Autodesk Inventor part; units mm, degrees
ref_plane "XZ Plane" through (0, 0, 0) normal (0, 1, 0) x (-1, 0, 0)
ref_plane "XY Plane" through (0, 0, 0) normal (0, 0, 1) x (1, 0, 0)
sketch "Sketch1" plane through (0, 0, 0) normal (0, 1, 0) x (-1, 0, 0)
  line L0 (0, 0) -> (60, 0)
  line L1 (60, 0) -> (60, -120)
  line L2 (60, -120) -> (0, -120)
  line L3 (0, -120) -> (0, 0)
  line L4 (60, 0) -> (0, -120) construction
  line L5 (60, -120) -> (0, 0) construction
  circle A0 centre (30, -60) radius 67.082
  line L6 (30, -120) -> (30, 7.082) construction
  line L7 (60, -60) -> (0, -60)
  line L8 (30, -60) -> (81.3878, -103.1195) construction
  line L9 (41.76, -45.985) -> (17.4815, -74.919) construction
  line L10 (-33, -36.9566) -> (-33, -83.0434)
  line L11 (93, -36.9566) -> (93, -83.0434)
  circle A1 centre (60, -110) radius 1.5
  circle A2 centre (70, -60) radius 12.5
  circle A3 centre (30, -100) radius 15
  circle A4 centre (84.4498, -80.8618) radius 1.5
  circle A5 centre (68.3022, -92.1394) radius 10
  circle A6 centre (30, -60) radius 15
  point P0 (60, -120)
  point P1 (60, 0)
  dimension "d0" = 120
  dimension "d25" = 60
  dimension "d27" = 50
  dimension "d38" = 63
  dimension "d39" = 63
  dimension "d50" = 3
  dimension "d51" = 10
  dimension "d52" = 25
  dimension "d53" = 40
  dimension "d54" = 30
  dimension "d55" = 40
  dimension "d56" = 20
  dimension "d57" = 50
  dimension "d58" = 30
extrude "Extrusion1" add sketch "Sketch1" along normal blind 3 contours L0 L1 A2 L7 A6 L3 | L3 A0 L10 | A0 L11 L1 A1 A5 A2 | L7 A6 A2 L1 A5 A1 L2 L3 | A2 L1 | L1 L7 A2 | A6 L7 | L7 A6 | L1 A2 L7 | A1 L1 | L1 A1 | A5 L1 | L1 A5 | A3 | A4
extrude "Extrusion3" cut sketch "Sketch1" along normal blind 10 contours A6 L7 | L7 A6 | A1 L1 | L1 A1 | A5 L1 | L1 A5 | A3 | A4
ref_plane "Work Plane5" through (-60, 0, -60) normal (0, 0, 1) x (1, 0, 0)
ref_plane "Work Plane6" through (-30, 0, 0) normal (1, 0, 0) x (0, 1, 0)
mirror "Mirror3" about plane through (-60, 0, -60) normal (0, 0, 1) of "Extrusion3"
mirror "Mirror4" about plane through (-30, 0, 0) normal (1, 0, 0) of "Extrusion3", "Mirror3"
sketch "Sketch10" plane through (0, 3, 0) normal (0, 1, 0) x (1, 0, 0)
  circle A0 centre (24.4498, 39.1382) radius 1.5
  circle A1 centre (8.3022, 27.8606) radius 10
  circle A2 centre (0, 10) radius 1.5
  circle A3 centre (24.4498, 80.8618) radius 1.5
  circle A4 centre (8.3022, 92.1394) radius 10
  circle A5 centre (0, 110) radius 1.5
  circle A6 centre (-84.4498, 39.1382) radius 1.5
  circle A7 centre (-68.3022, 27.8606) radius 10
  circle A8 centre (-60, 10) radius 1.5
  circle A9 centre (-30, 20) radius 15
  circle A10 centre (-84.4498, 80.8618) radius 1.5
  circle A11 centre (-68.3022, 92.1394) radius 10
  circle A12 centre (-60, 110) radius 1.5
  circle A13 centre (-30, 100) radius 15
  circle A14 centre (-30, 60) radius 15
  line L0 (0, 120) -> (-60, 120)
  arc A15 (-60, 120) -> (-93, 83.0434) centre (-30, 60) ccw
  line L1 (-93, 83.0434) -> (-93, 36.9566)
  arc A16 (-93, 36.9566) -> (-60, 0) centre (-30, 60) ccw
  line L2 (-60, 0) -> (0, 0)
  arc A17 (0, 0) -> (33, 36.9566) centre (-30, 60) ccw
  line L3 (33, 36.9566) -> (33, 83.0434)
  arc A18 (33, 83.0434) -> (0, 120) centre (-30, 60) ccw
sketch "Sketch14" plane through (0, 3, 0) normal (0, 1, 0) x (1, 0, 0)
  circle A0 centre (-89, 70) radius 1.5
  circle A1 centre (-89, 50) radius 1.5
  line L0 (-93, 83.0434) -> (-93, 36.9566)
  line L1 (63.1517, 60) -> (-123.1517, 60)
  point P0 (0, 0)
  dimension "d75" = 3
  dimension "d76" = 3
  dimension "d77" = 4
  dimension "d78" = 4
  dimension "d79" = 10
  dimension "d80" = 10
extrude "Extrusion6" cut sketch "Sketch14" against normal blind 10
properties part number "Drone_plate_3"
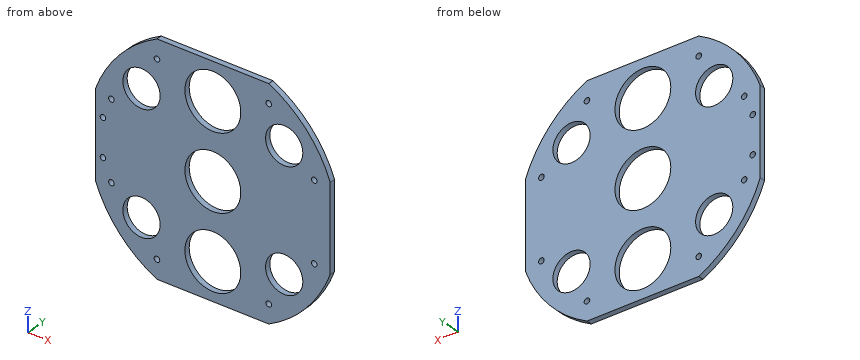
Source: CAD feature listing. Evaluate the final solid. Frame: model axes, mm. Round coordinates to 2 decimals unless told otherwise and drop trailing zeros. Loops run counter-clockwise (first coordinate to the right, second up) from the corner with the lowest first, then second, coordinate; pieces in that order, holes last. Notation, with made-up numbers: M 67,7 L 126,7 A7 cw 126,17 Z; hole C 44,29 d1. An arc over 180 degrees is marked long. Use a Markdown table: item, result. Add a question column.
1. Section query B-B on z = -110. Return the cut outline in (x, y).
2. Line query: line 1 (Z direction, x = -39, y = 0.4); line 2 (X direction, y = 1.45, z = -110); line 3 (Z direction, x = -31, y = 2.7). Output: solid intervals per line, ascending.
3. Section query D-D on y = 1.15. Give the number of separate pieces and of enclosed holes in the cut face, then the cut area to 3 significant figures.
4. Section query A-A on x = -30. Return the cut outline in (y, z), then the cut area to 3 significant figures.
5. Contact query for flat-ended pins moving along their axis: P1, Ø2.5, axis at x = -60, z = -110, coming from the -Y side; P2, Ø1, axis at x = -65.5, y = 1, coming from the -Z side. Output: stop coordinate, or through.
6. Section query C-C on z = -70. Return the cut outline in (x, y).
Reported:
| question | item | result |
|---|---|---|
| 1 | outline | M -74.72,0 L -61.5,0 L -61.5,3 L -74.72,3 Z; M -58.5,0 L -41.18,0 L -41.18,3 L -58.5,3 Z; M -18.82,0 L -1.5,0 L -1.5,3 L -18.82,3 Z; M 1.5,0 L 14.72,0 L 14.72,3 L 1.5,3 Z |
| 2 | line 1 | z = -120 to -112, -88 to -72, -48 to -32, -8 to 0 |
| 2 | line 2 | x = -74.72 to -61.5, -58.5 to -41.18, -18.82 to -1.5, 1.5 to 14.72 |
| 2 | line 3 | z = -120 to -114.97, -85.03 to -74.97, -45.03 to -34.97, -5.03 to 0 |
| 3 | separate pieces | 1 |
| 3 | enclosed holes | 17 |
| 3 | area | 9,860 mm² |
| 4 | outline | M 0,-120 L 3,-120 L 3,-115 L 0,-115 Z; M 0,-85 L 3,-85 L 3,-75 L 0,-75 Z; M 0,-45 L 3,-45 L 3,-35 L 0,-35 Z; M 0,-5 L 3,-5 L 3,0 L 0,0 Z |
| 4 | area | 90.0 mm² |
| 5 | P1 | passes through |
| 5 | P2 | stops at z = -117.23 |
| 6 | outline | M -93,0 L -90.5,0 L -90.5,3 L -93,3 Z; M -87.5,0 L -41.18,0 L -41.18,3 L -87.5,3 Z; M -18.82,0 L 33,0 L 33,3 L -18.82,3 Z |
